Model file for the job. Use its own axes, mm. A direction names the side the tool comes from. Give positions to 0.01 mm unless a question says otherwise; leave off trailing zeros. Order: outer loops, then holes, each group sorted by start corner. A loop starts at its lowest first (then second) coordinate and runs counter-clockwise, first axis right, second up. Notation, with made-up numbers: (50.25, 5) - (100.25, 5) arc R16 cw to (100.25, 34) - close; hole circle Ø10 at (74, 37). An arc over 180 degrees is marked (long way). Return JSON: item names as keys, results as strings. Group by question number.
from build123d import *

# Parameters (mm, degrees)
CHAMFER1_SIZE = 1.27
FILLET1_R     = 0.762


with BuildPart() as part:
    # Sketch1 → Base-Revolve (revolve)
    with BuildSketch(Plane.XY, mode=Mode.PRIVATE) as base_revolve_sk:
        Polygon((0, 35.56), (0, 48.26), (7.62, 48.26), (7.62, 50.8), (48.26, 50.8), (50.8, 48.26), (58.42, 48.26), (58.42, 63.5), (71.12, 63.5), (71.12, 42.416108007), (75.319090909, 42.416108007), (79.129090909, 45.72), (127, 45.72), (127, 35.56), (83.82, 35.56), (81.915, 33.02), (63.5, 33.02), (63.5, 30.48), (38.1, 30.48), (38.1, 38.1), (10.16, 38.1), (10.16, 35.56), align=None)
    revolve(base_revolve_sk.sketch.rotate(Axis((0, 0, 0), (1, 0, 0)), 90), axis=Axis((0, 0, 0), (1, 0, 0)))

    # Chamfer1
    chamfer1_edges = [part.edges().sort_by_distance(p)[0] for p in [
        (0, 0, -35.56),
        (7.62, 0, -50.8),
        (58.42, 0, -63.5),
        (71.12, 0, -63.5),
        (127, 0, -45.72),
        (127, 0, -35.56),
        (38.1, 0, -30.48),
    ]]
    chamfer(chamfer1_edges, length=CHAMFER1_SIZE)

    # Fillet1
    fillet1_edges = [part.edges().sort_by_distance(p)[0] for p in [
        (0, 0, -48.26),
    ]]
    fillet(fillet1_edges, radius=FILLET1_R)


solid = part.part
(1) Drill centre lines: L1, parallel to Y at x = 72.5, z = 0; L2, parallel to Z at x = 85, y = -0.5; L3, parallel to Y at x = 67, z = 0. Where is each one in solid material? Low to high.
(2) Slice it at A-A (x = 23.5). Give the cut face in (y, z).
(3) Pull direction Z, two halves, no side cores. Call faces 5 (the face through (127, -33, -17)), 6 (the face through (63.5, 10, 29)), 7 (the face through (5.653, 34.714, -7.709)), 8 (the face through (28.851, 30.911, -40.313)): released by +Z, released by -Z, zero draft, split by the parting line, or undercut.
(4) Drop flat-ended pins along their axis: pin 1 Ø23 at (y, z) = (-17.5, 6) entering from +X; pin 2 Ø3 at (y, z) = (33.5, 9.5) entering from -X; pin 3 Ø4 at (y, z) = (49.5, -42.5) entering from -X; pin 4 Ø1.5 at (x, z) = (103, -40.5) entering from -Y. Give the stop position or say it passes through.
(5) Slice it at B-B (x = 115.5). Give the cut face in (y, z), and give its area (3 significant figures).
(6) 3-axis set-ups, long thin cutter, end or side, ignore diameter. For faces 1 (the face through (71.12, 13, 41)), 2 (the face through (4.24, -14.5, 46.03)), 3 (the face through (0, 27.9, -24.4)), 4 (the face through (72.579, 29.294, 15.237)): which of +Z, -Z, +X, -X, +Y, -Y reach the whole face in a straight line?
Result set:
{
 "1": {"L1": "y = -42.42 to -33.02, 33.02 to 42.42", "L2": "z = -45.72 to -35.56, 35.56 to 45.72", "L3": "y = -63.5 to -33.02, 33.02 to 63.5"},
 "2": {"outline": "circle Ø101.6 at (0, 0); hole circle Ø76.2 at (0, 0)"},
 "3": {"face 5": "zero draft", "face 6": "undercut", "face 7": "undercut", "face 8": "split by the parting line"},
 "4": {"pin 1": "passes through", "pin 2": "stops at x = 0.51", "pin 3": "stops at x = 59.43", "pin 4": "stops at y = -22.59"},
 "5": {"outline": "circle Ø91.44 at (0, 0); hole circle Ø71.12 at (0, 0)", "area": "2,590 mm²"},
 "6": {"face 1": "none", "face 2": "-X", "face 3": "+Z, -Z, -X, +Y, -Y", "face 4": "+X"}
}
